```python
from build123d import *

# Parameters (mm, degrees)
EXTRUDE_1_DEPTH = 100


with BuildPart() as part:
    # Эскиз1 → Бобышка-Вытянуть1 (new body)
    with BuildSketch(Plane.XY):
        with BuildLine():
            Line((311.090891371, 325.050300163), (319.788031344, 324.810224137))
            ThreePointArc((319.788031344, 324.810224137), (319.867529895, 324.824333608), (319.934971402, 324.868726626))
            Line((319.934971402, 324.868726626), (320.131212385, 325.064967609))
            Line((320.131212385, 325.064967609), (323.201898914, 325.064967609))
            Line((323.201898914, 325.064967609), (324.141129398, 325.607232582))
            ThreePointArc((324.141129398, 325.607232582), (324.241129398, 325.634027502), (324.341129398, 325.607232582))
            Line((324.341129398, 325.607232582), (325.280359883, 325.064967609))
            Line((325.280359883, 325.064967609), (328.141129398, 325.064967609))
            ThreePointArc((328.141129398, 325.064967609), (328.282550755, 325.123546253), (328.341129398, 325.264967609))
            Line((328.341129398, 325.264967609), (328.341129398, 335.660147982))
            ThreePointArc((328.341129398, 335.660147982), (327.90178957, 336.720808154), (326.841129398, 337.160147982))
            Line((326.841129398, 337.160147982), (326.751018387, 337.160147982))
            ThreePointArc((326.751018387, 337.160147982), (326.609597031, 337.101569338), (326.551018387, 336.960147982))
            Line((326.551018387, 336.960147982), (326.551018387, 336.898541414))
            ThreePointArc((326.551018387, 336.898541414), (326.50335276, 336.768948826), (326.383075998, 336.701127358))
            ThreePointArc((326.383075998, 336.701127358), (326.273318939, 336.619532133), (326.27674616, 336.482811079))
            Line((326.27674616, 336.482811079), (326.447277251, 336.173129229))
            ThreePointArc((326.447277251, 336.173129229), (326.451076485, 336.109455402), (326.40409571, 336.066309172))
            Line((326.40409571, 336.066309172), (326.066600192, 335.962234792))
            ThreePointArc((326.066600192, 335.962234792), (325.96870237, 335.864988428), (325.99301838, 335.729159231))
            Line((325.99301838, 335.729159231), (326.209580677, 335.450169137))
            ThreePointArc((326.209580677, 335.450169137), (326.223272021, 335.387868756), (326.183601656, 335.337918255))
            Line((326.183601656, 335.337918255), (325.866171063, 335.182285611))
            ThreePointArc((325.866171063, 335.182285611), (325.784195666, 335.067661744), (325.834812154, 334.936145328))
            Line((325.834812154, 334.936145328), (326.08754177, 334.719229546))
            ThreePointArc((326.08754177, 334.719229546), (326.113257599, 334.657577201), (326.079055863, 334.600196396))
            Line((326.079055863, 334.600196396), (325.798110573, 334.421326447))
            ThreePointArc((325.798110573, 334.421326447), (325.729347274, 334.298199433), (325.794435238, 334.173090641))
            Line((325.794435238, 334.173090641), (326.083482656, 333.976799787))
            ThreePointArc((326.083482656, 333.976799787), (326.132220057, 333.889114864), (326.090713273, 333.797784875))
            Line((326.090713273, 333.797784875), (325.834605364, 333.591823003))
            ThreePointArc((325.834605364, 333.591823003), (325.779589072, 333.464527861), (325.853621615, 333.347267346))
            Line((325.853621615, 333.347267346), (326.141686948, 333.18153099))
            ThreePointArc((326.141686948, 333.18153099), (326.178703219, 333.122900733), (326.151195073, 333.059253162))
            Line((326.151195073, 333.059253162), (325.892212173, 332.850979224))
            ThreePointArc((325.892212173, 332.850979224), (325.837195882, 332.723684082), (325.911228424, 332.606423567))
            Line((325.911228424, 332.606423567), (326.199293757, 332.440687211))
            ThreePointArc((326.199293757, 332.440687211), (326.236310028, 332.382056954), (326.208801882, 332.318409383))
            Line((326.208801882, 332.318409383), (325.949818982, 332.110135445))
            ThreePointArc((325.949818982, 332.110135445), (325.894802691, 331.982840302), (325.968835233, 331.865579788))
            Line((325.968835233, 331.865579788), (326.256900566, 331.699843432))
            ThreePointArc((326.256900566, 331.699843432), (326.293916837, 331.641213174), (326.266408691, 331.577565603))
            Line((326.266408691, 331.577565603), (326.007425791, 331.369291665))
            ThreePointArc((326.007425791, 331.369291665), (325.9524095, 331.241996523), (326.026442042, 331.124736008))
            Line((326.026442042, 331.124736008), (326.314507375, 330.958999652))
            ThreePointArc((326.314507375, 330.958999652), (326.351523646, 330.900369395), (326.3240155, 330.836721824))
            Line((326.3240155, 330.836721824), (326.0650326, 330.628447886))
            ThreePointArc((326.0650326, 330.628447886), (326.010016309, 330.501152743), (326.084048851, 330.383892229))
            Line((326.084048851, 330.383892229), (326.372114184, 330.218155873))
            ThreePointArc((326.372114184, 330.218155873), (326.409130455, 330.159525616), (326.381622309, 330.095878044))
            Line((326.381622309, 330.095878044), (326.12263941, 329.887604106))
            ThreePointArc((326.12263941, 329.887604106), (326.067623118, 329.760308964), (326.14165566, 329.643048449))
            Line((326.14165566, 329.643048449), (326.429720993, 329.477312094))
            ThreePointArc((326.429720993, 329.477312094), (326.466737264, 329.418681836), (326.439229119, 329.355034265))
            Line((326.439229119, 329.355034265), (326.180246219, 329.146760327))
            ThreePointArc((326.180246219, 329.146760327), (326.125229927, 329.019465185), (326.199262469, 328.90220467))
            Line((326.199262469, 328.90220467), (326.487327802, 328.736468314))
            ThreePointArc((326.487327802, 328.736468314), (326.524344073, 328.677838057), (326.496835928, 328.614190486))
            Line((326.496835928, 328.614190486), (326.237853028, 328.405916548))
            ThreePointArc((326.237853028, 328.405916548), (326.182836736, 328.278621405), (326.256869279, 328.161360891))
            Line((326.256869279, 328.161360891), (326.640868299, 327.940429765))
            ThreePointArc((326.640868299, 327.940429765), (326.71425909, 327.867204665), (326.741129398, 327.767074201))
            Line((326.741129398, 327.767074201), (326.741129398, 326.710147982))
            ThreePointArc((326.741129398, 326.710147982), (326.682550755, 326.568726626), (326.541129398, 326.510147982))
            Line((326.541129398, 326.510147982), (321.941129398, 326.510147982))
            ThreePointArc((321.941129398, 326.510147982), (321.799708042, 326.568726626), (321.741129398, 326.710147982))
            Line((321.741129398, 326.710147982), (321.741129398, 327.486517476))
            ThreePointArc((321.741129398, 327.486517476), (321.767999707, 327.586647941), (321.841390498, 327.659873041))
            Line((321.841390498, 327.659873041), (322.202552193, 327.867664872))
            ThreePointArc((322.202552193, 327.867664872), (322.276584735, 327.984925387), (322.221568443, 328.112220529))
            Line((322.221568443, 328.112220529), (321.962585543, 328.320494467))
            ThreePointArc((321.962585543, 328.320494467), (321.935077398, 328.384142038), (321.972093669, 328.442772296))
            Line((321.972093669, 328.442772296), (322.260159002, 328.608508652))
            ThreePointArc((322.260159002, 328.608508652), (322.334191544, 328.725769166), (322.279175253, 328.853064309))
            Line((322.279175253, 328.853064309), (322.020192353, 329.061338247))
            ThreePointArc((322.020192353, 329.061338247), (321.992684207, 329.124985818), (322.029700478, 329.183616075))
            Line((322.029700478, 329.183616075), (322.317765811, 329.349352431))
            ThreePointArc((322.317765811, 329.349352431), (322.391798353, 329.466612946), (322.336782062, 329.593908088))
            Line((322.336782062, 329.593908088), (322.077799162, 329.802182026))
            ThreePointArc((322.077799162, 329.802182026), (322.050291016, 329.865829597), (322.087307287, 329.924459854))
            Line((322.087307287, 329.924459854), (322.37537262, 330.09019621))
            ThreePointArc((322.37537262, 330.09019621), (322.449405162, 330.207456725), (322.394388871, 330.334751867))
            Line((322.394388871, 330.334751867), (322.135405971, 330.543025805))
            ThreePointArc((322.135405971, 330.543025805), (322.107897825, 330.606673377), (322.144914096, 330.665303634))
            Line((322.144914096, 330.665303634), (322.432979429, 330.83103999))
            ThreePointArc((322.432979429, 330.83103999), (322.507011971, 330.948300504), (322.45199568, 331.075595647))
            Line((322.45199568, 331.075595647), (322.19301278, 331.283869585))
            ThreePointArc((322.19301278, 331.283869585), (322.165504634, 331.347517156), (322.202520905, 331.406147413))
            Line((322.202520905, 331.406147413), (322.490586238, 331.571883769))
            ThreePointArc((322.490586238, 331.571883769), (322.564618781, 331.689144284), (322.509602489, 331.816439426))
            Line((322.509602489, 331.816439426), (322.250619589, 332.024713364))
            ThreePointArc((322.250619589, 332.024713364), (322.223111443, 332.088360935), (322.260127715, 332.146991193))
            Line((322.260127715, 332.146991193), (322.548193048, 332.312727548))
            ThreePointArc((322.548193048, 332.312727548), (322.62222559, 332.429988063), (322.567209298, 332.557283205))
            Line((322.567209298, 332.557283205), (322.308226398, 332.765557144))
            ThreePointArc((322.308226398, 332.765557144), (322.280718253, 332.829204715), (322.317734524, 332.887834972))
            Line((322.317734524, 332.887834972), (322.605799857, 333.053571328))
            ThreePointArc((322.605799857, 333.053571328), (322.679832399, 333.170831842), (322.624816107, 333.298126985))
            Line((322.624816107, 333.298126985), (322.365833207, 333.506400923))
            ThreePointArc((322.365833207, 333.506400923), (322.338325062, 333.570048494), (322.375341333, 333.628678751))
            Line((322.375341333, 333.628678751), (322.663406666, 333.794415107))
            ThreePointArc((322.663406666, 333.794415107), (322.737622, 333.914334818), (322.678209577, 334.042236409))
            Line((322.678209577, 334.042236409), (322.411350306, 334.241512209))
            ThreePointArc((322.411350306, 334.241512209), (322.381512328, 334.301278508), (322.411743655, 334.360846808))
            Line((322.411743655, 334.360846808), (322.679910814, 334.558359061))
            ThreePointArc((322.679910814, 334.558359061), (322.740171486, 334.685745276), (322.666950969, 334.806150228))
            Line((322.666950969, 334.806150228), (322.361978717, 334.984967527))
            ThreePointArc((322.361978717, 334.984967527), (322.326134471, 335.037730965), (322.344422849, 335.098840094))
            Line((322.344422849, 335.098840094), (322.581141078, 335.36094538))
            ThreePointArc((322.581141078, 335.36094538), (322.615495018, 335.494589107), (322.525103363, 335.598849299))
            Line((322.525103363, 335.598849299), (322.196285999, 335.727743993))
            ThreePointArc((322.196285999, 335.727743993), (322.152645383, 335.774265892), (322.161171245, 335.837480605))
            Line((322.161171245, 335.837480605), (322.354269218, 336.133617186))
            ThreePointArc((322.354269218, 336.133617186), (322.366051346, 336.274044313), (322.25526952, 336.361141866))
            Line((322.25526952, 336.361141866), (322.106867151, 336.386946327))
            ThreePointArc((322.106867151, 336.386946327), (321.988073119, 336.455250544), (321.941129398, 336.58398972))
            Line((321.941129398, 336.58398972), (321.941129398, 336.960147982))
            ThreePointArc((321.941129398, 336.960147982), (321.882550755, 337.101569338), (321.741129398, 337.160147982))
            Line((321.741129398, 337.160147982), (321.641129398, 337.160147982))
            ThreePointArc((321.641129398, 337.160147982), (320.580469227, 336.720808154), (320.141129398, 335.660147982))
            Line((320.141129398, 335.660147982), (320.141129398, 327.928017713))
            ThreePointArc((320.141129398, 327.928017713), (320.179892433, 327.809684958), (320.281155808, 327.737221569))
            ThreePointArc((320.281155808, 327.737221569), (320.624342386, 327.177574585), (320.117425076, 326.760421597))
            Line((320.117425076, 326.760421597), (309.643319038, 327.04954903))
            ThreePointArc((309.643319038, 327.04954903), (309.498343785, 326.992984419), (309.437800337, 326.849625185))
            Line((309.437800337, 326.849625185), (309.437800337, 326.749652848))
            ThreePointArc((309.437800337, 326.749652848), (309.919246841, 325.564272159), (311.090891371, 325.050300163))
        make_face()
    extrude(amount=EXTRUDE_1_DEPTH)


solid = part.part
```
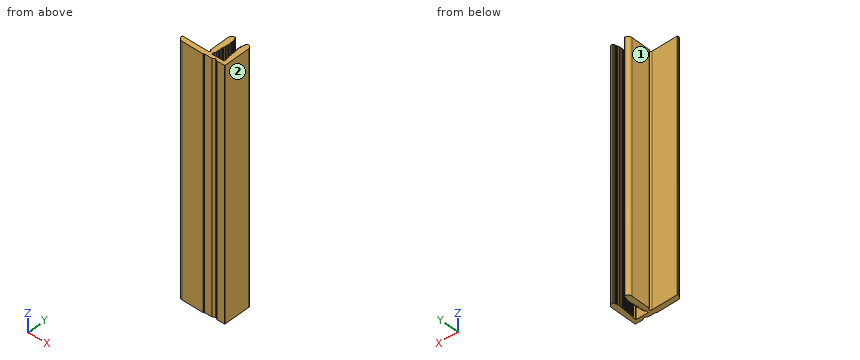
CAD build for the part. Positions are in the model's coordinates, mm. Face numbers are marked on the shaded views. A direction names the side the tool comes from. Round coordinates to 2 decimals unless told otherwise and drop trailing zeros. Loops run counter-clockwise (first coordinate to the right, second up) from the corner with the lowest first, then second, coordinate; pieces in that order, holes last. Notation, with made-up numbers: M -1.5,45 L 14.5,45 A31 ccw 14.5,75 Z; hole C 77.5,83 d6. An arc over 180 degrees is marked long. Use a Markdown table: item, result. Add a question column.
(1) Drill centre lines: line 1 (X direction, y = 333.75, z = 44); line 2 (X direction, y = 334, z = 95.5); line 3 (Y direction, x = 321.5, z = 57). Where is each one in solid material? Low to high.
(2) Flat gauge pins, fed straight in: pin 1 (5 mm diameter, centred on x = 324, z = 59, fed in from +Y); pin 2 (4 mm diameter, centred on y = 332.5, z = 61, fed in from -X); pin 3 (2.5 mm diameter, centred on x = 322, z = 64.5, fed in from -Y); pin 4 (2 mm diameter, centred on x = 318.5, z = 59, fed in from +Y). Where does each tip first touch, or does it go through?
(3) Which spindle directions (+Z, -Z, +X, -X, +Y, -Y) get a long thin tool onto all of the face, cutting with end or side? Do the marked faces 1 and 2. Say none if no direction does.
(4) Cut at A-A (x = 312.25). Give the cut face in (y, z), and give its area (3 significant figures).
Geometry says:
| question | item | result |
|---|---|---|
| 1 | line 1 | x = 320.14 to 322.59, 326.03 to 328.34 |
| 1 | line 2 | x = 320.14 to 322.72, 326.05 to 328.34 |
| 1 | line 3 | y = 325.06 to 337.15 |
| 2 | pin 1 | stops at y = 337.16 |
| 2 | pin 2 | stops at x = 320.14 |
| 2 | pin 3 | stops at y = 325.06 |
| 2 | pin 4 | stops at y = 326.83 |
| 3 | face 1 | +Z, -Z, -X, +Y |
| 3 | face 2 | +Z, -Z, +X, +Y, -Y |
| 4 | outline | M 325.02,0 L 326.98,0 L 326.98,100 L 325.02,100 Z |
| 4 | area | 196 mm² |
